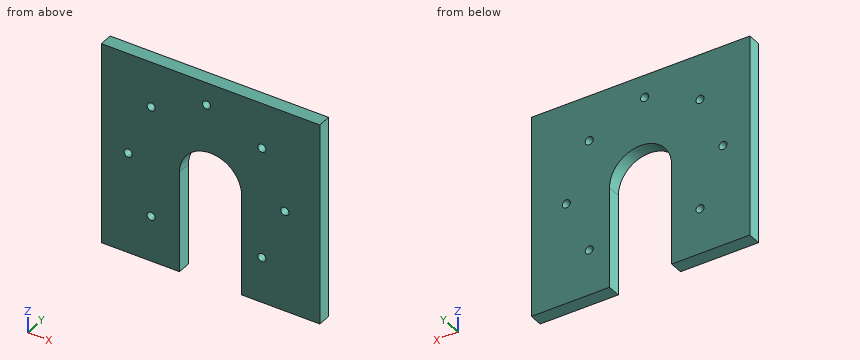
```python
from build123d import *

# Parameters (mm, degrees)
F0_W             = 650
F0_H             = 600
F1_DEPTH         = 40
F3_DEPTH         = 40.001
F4_R             = 12
F5_DEPTH         = 40.001
F5_COPIES_COUNT  = 4
F5_COPIES_ANGLE  = 135
F5_COPIES1_COUNT = 4
F5_COPIES1_ANGLE = 135


# Not quite as in the source:
# - a pattern or mirror of a feature is missing from the dataset's text; its kind, count and spacing are read off the source's solid


with BuildPart() as f1:
    # F0 (on Front) → F1 (new body)
    with BuildSketch(Plane.XZ):
        with Locations((12.1025014669, -20.5410706814)):
            Rectangle(F0_W, F0_H)
    extrude(amount=F1_DEPTH)

    # F2 (on face) → F3 (cut, through all)
    with BuildSketch(Plane.XZ.offset(40)):
        with BuildLine():
            Line((-80.3974985331, -20.5410706814), (-80.3974985331, -320.5410706814))
            Line((-80.3974985331, -320.5410706814), (104.6025014669, -320.5410706814))
            Line((104.6025014669, -320.5410706814), (104.6025014669, -20.5410706814))
            ThreePointArc((104.6025014669, -20.5410706814), (12.1025014669, 71.9589293186), (-80.3974985331, -20.5410706814))
        make_face()
    extrude(amount=-F3_DEPTH, mode=Mode.SUBTRACT)

    # F4 (on face) → F5 (cut, through all)
    with BuildSketch(Plane.XZ.offset(40)):
        with Locations((0, 212.4589293186)):
            Circle(F4_R)
    f5 = extrude(amount=-F5_DEPTH, mode=Mode.SUBTRACT)

    # F5_copies: F5 ×4 about axis
    f5_copies_axis = Axis((0, 0, -20.541071), (0, 1, 0))
    for i in range(1, F5_COPIES_COUNT):
        add(f5.rotate(f5_copies_axis, i * F5_COPIES_ANGLE / (F5_COPIES_COUNT - 1)), mode=Mode.SUBTRACT)

    # F5_copies1: F5 ×4 about axis
    f5_copies1_axis = Axis((0, 0, -20.541071), (0, -1, 0))
    for i in range(1, F5_COPIES1_COUNT):
        add(f5.rotate(f5_copies1_axis, i * F5_COPIES1_ANGLE / (F5_COPIES1_COUNT - 1)), mode=Mode.SUBTRACT)


solid = f1.part
```
Could you check a few things on this model? Use its own coordinates, in mm. Give positions to 0.01 mm unless a question says otherwise; leave off trailing zeros. Order: outer loops, then holes, each group sorted by start corner. A loop starts at its lowest first (then second) coordinate and runs counter-clockwise, first axis right, second up.
Q1. Suppose I cut it at C-C, the plane y = -11.5. Write out the boundary of the cut face in (x, z), and give its area (3 significant figures).
Q2. Suppose I cut it at A-A, the plane z = -270. Write out the boundary of the cut face in (x, y), and give its area (3 significant figures).
Q3. If I drill on line 1 along X through (y, z) = (-19.5, -59.5); line 2 along X through (y, z) = (-17.5, -29.5); line 3 along X through (y, z) = (-14, -25.5), over which ranges is the centre line in solid material (lowest first)?
Q4. Suppose I cut it at B-B, the plane x = -233. Write out the boundary of the cut face in (y, z), and give its area (3 significant figures).
Solution:
1. outline: (-312.9, -320.54) - (-80.4, -320.54) - (-80.4, -20.54) arc R92.5 cw to (104.6, -20.54) - (104.6, -320.54) - (337.1, -320.54) - (337.1, 279.46) - (-312.9, 279.46) - close; hole circle Ø24 at (-233, -20.54); hole circle Ø24 at (-164.76, -185.3); hole circle Ø24 at (-164.76, 144.21); hole circle Ø24 at (0, 212.46); hole circle Ø24 at (164.76, -185.3); hole circle Ø24 at (164.76, 144.21); hole circle Ø24 at (233, -20.54)
1. area: 318,000 mm2
2. outline: (-312.9, -40) - (-80.4, -40) - (-80.4, 0) - (-312.9, 0) - close; (104.6, -40) - (337.1, -40) - (337.1, 0) - (104.6, 0) - close
2. area: 18,600 mm2
3. line 1: x = -312.9 to -80.4, 104.6 to 337.1
3. line 2: x = -312.9 to -240.98, -225.02 to -80.4, 104.6 to 225.02, 240.98 to 337.1
3. line 3: x = -312.9 to -243.93, -222.07 to -80.4, 104.6 to 222.07, 243.93 to 337.1
4. outline: (-40, -320.54) - (0, -320.54) - (0, -32.54) - (-40, -32.54) - close; (-40, -8.54) - (0, -8.54) - (0, 279.46) - (-40, 279.46) - close
4. area: 23,000 mm2
